```python
from build123d import *

# Parameters (mm, degrees)
SKETCH1_R           = 14.2875
BOSS_EXTRUDE1_DEPTH = 7.62
CUT_EXTRUDE1_DEPTH  = 8.62
FILLET1_R           = 1.27


with BuildPart() as part:
    # Sketch1 → Boss-Extrude1 (new body)
    with BuildSketch(Plane(origin=(0, 0, 0), x_dir=(1, 0, 0), z_dir=(0, 1, 0))):
        with BuildLine():
            Line((7.49794353, -57.888099751), (21.467701489, -5.752253277))
            ThreePointArc((21.467701489, -5.752253277), (17.632277988, 13.52972276), (0, 22.225))
            ThreePointArc((0, 22.225), (-13.52972276, 17.632277988), (-21.467701489, 5.752253277))
            Line((-21.467701489, 5.752253277), (-35.437459449, -46.383593197))
            ThreePointArc((-35.437459449, -46.383593197), (-19.722011237, -73.603547963), (7.49794353, -57.888099751))
        make_face()
        with Locations((-13.969757959, -52.135846474)):
            Circle(SKETCH1_R, mode=Mode.SUBTRACT)
        Circle(SKETCH1_R, mode=Mode.SUBTRACT)
    extrude(amount=BOSS_EXTRUDE1_DEPTH)

    # Sketch2 → Cut-Extrude1 (cut, through all)
    with BuildSketch(Plane(origin=(0, 7.62, 0), x_dir=(1, 0, 0), z_dir=(0, 1, 0))):
        Polygon((-20.393980488, -14.77508138), (-3.03503134, -35.86140715), (-24.502732829, -30.109153872), align=None)
        Polygon((-10.93472662, -16.274439324), (10.532974869, -22.026692602), (6.424222528, -37.360765094), align=None)
    extrude(amount=-CUT_EXTRUDE1_DEPTH, mode=Mode.SUBTRACT)

    # Fillet1
    fillet1_edges = [part.edges().sort_by_distance(p)[0] for p in [
        (-24.502732829, 3.81, 30.109153872),
        (-20.393980488, 3.81, 14.77508138),
        (-3.03503134, 3.81, 35.86140715),
        (6.424222528, 3.81, 37.360765094),
        (-10.93472662, 3.81, 16.274439324),
        (10.532974869, 3.81, 22.026692602),
    ]]
    fillet(fillet1_edges, radius=FILLET1_R)


solid = part.part
```
The model under review builds one solid part; all positions refer to its coordinate system, in mm. A direction names the side the tool comes from. Give positions to 0.01 mm unless a question says otherwise; leave off trailing zeros. Write each loop counter-clockwise with the first axis right and the second up, starting at its lowest first coordinate (ties: lowest second). Pieces come first, ordered by that corner, then holes.
(1) Consider section C-C, the plane x = 12.5. Give the boundary of the cut face in (y, z), and give its area (3 significant figures).
(2) To check wall thickness, follow L1, parallel to X at y = 0.75, z = 23; L2, parallel to X at y = 1.5, z = 43; L3, parallel to Z at x = -5.5, y = 4.5. State the ranges of each line that lie inside material, in increasing order.
(3) Tool access review of faces 5 (the cylindrical face through (-20.09, 3.76, 16.25)), 6 (the flat face through (-7, 7.62, 25)): name each direction out of +Z, -Z, +X, -X, +Y, -Y from which nothing blocks a thin tool from reaching the whole face with its end or side.
(4) Consider section D-D, the plane y = 2.25. Give the number of separate pieces and of enclosed holes in the cut face, and give its area (3 significant figures).
(5) The part is to be moulded in two halves that separate along X. For faces 1 (the cylindrical face through (-17.067, 3.757, 66.084)), 2 (the flat face through (-7, 0, 25)), 3 (the flat face through (14.385, 3.757, 32.185)), 4 (the cylindrical face through (-20.193, 3.757, 73.472)), say which applies: released by +X, released by -X, zero draft, split by the parting line, or undercut.
(6) Consider section A-A, the plane x = -17. Give the boundary of the cut face in (y, z), and give its area (3 significant figures).
(7) For P1, Ø1.5, axis at x = -13, y = 6.5, coming from the +Z side; P2, Ø2, axis at x = -9, y = 6.5, coming from the +Z side; P3, Ø1.5, axis at x = -16, y = 4.5, coming from the +Z side, all flat-tipped, find the tip position at first contact; note any pin that passes through.
(8) Consider section B-B, the plane z = 0. Give the boundary of the cut face in (x, y) (1 decimal).
Returned:
1. outline: (0, -18.38) - (7.62, -18.38) - (7.62, -6.92) - (0, -6.92) - close; (0, 6.92) - (7.62, 6.92) - (7.62, 39.22) - (0, 39.22) - close
1. area: 333 mm2
2. L1: x = -29.17 to -22.6, -13.62 to -5.4, 10.25 to 16.85
2. L2: x = -34.53 to -24.95, -2.98 to 11.49
2. L3: z = -21.53 to -13.19, 13.19 to 17.73, 22.88 to 32.87, 34.35 to 40.63, 63.64 to 72.68
3. face 5: +Y, -Y
3. face 6: +Z, -Z, +X, -X, +Y
4. separate pieces: 1
4. enclosed holes: 4
4. area: 2,320 mm2
5. face 1: undercut
5. face 2: zero draft
5. face 3: released by +X
5. face 4: split by the parting line
6. outline: (0, -14.32) - (7.62, -14.32) - (7.62, 18.9) - (0, 18.9) - close; (0, 32.12) - (7.62, 32.12) - (7.62, 38.17) - (0, 38.17) - close; (0, 66.1) - (7.62, 66.1) - (7.62, 74.15) - (0, 74.15) - close
6. area: 361 mm2
7. P1: stops at z = 74.36
7. P2: stops at z = 74
7. P3: stops at z = 74.32
8. outline: (-23, 0) - (-14.3, 0) - (-14.3, 7.6) - (-23, 7.6) - close; (14.3, 0) - (22.2, 0) - (22.2, 7.6) - (14.3, 7.6) - close
